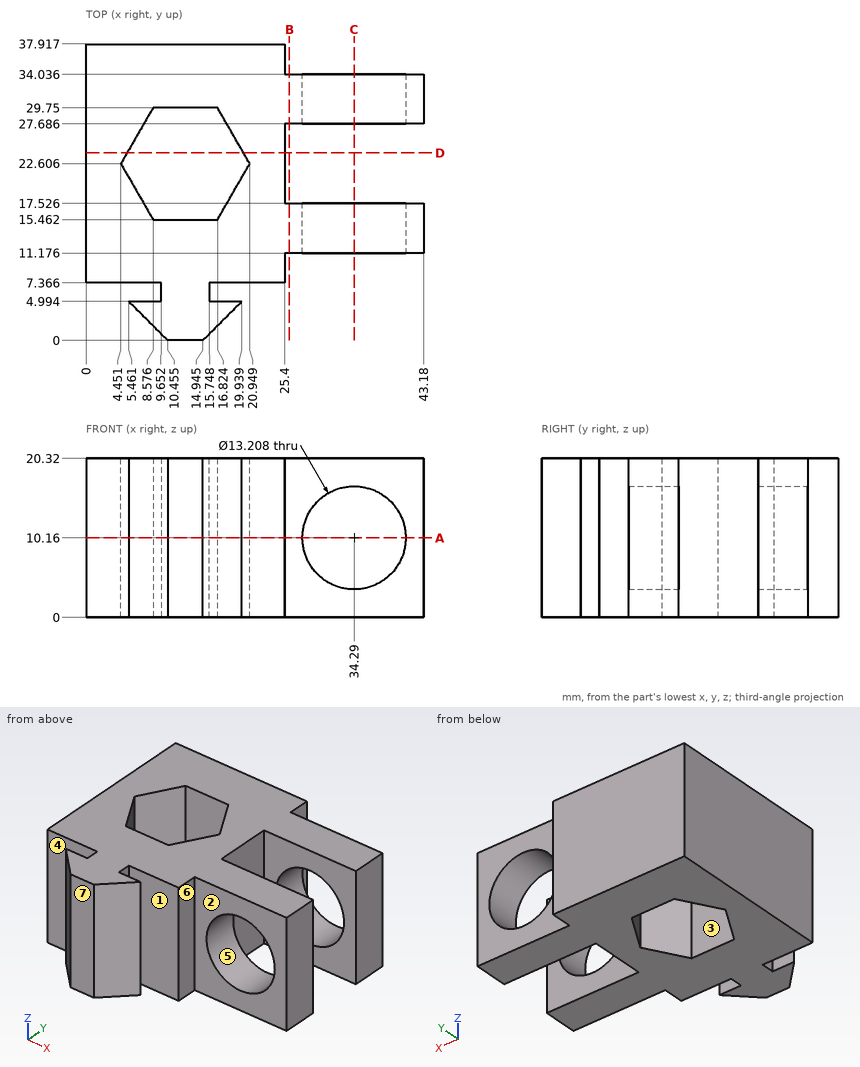
Here's the drawing with two shaded views (mm, measured from the low corner). I have some questions. A direction names the side the tool comes from. Give positions to 0.01 mm unless a question says otherwise; leave off trailing zeros. Order: outer loops, then holes, each group sorted by start corner. A loop starts at its lowest first (then second) coordinate and runs counter-clockwise, first axis right, second up. Notation, with made-up numbers: M -19.5,37 L 33.5,37 A21 ccw 33.5,44 Z; hole C 15.25,11.25 d5. An arc over 180 degrees is marked long. Answer as a JSON object with one key per item and string values. Group by question number.
1) Suppose I cut it at B-B, the plane x = 26. Write out the boundary of the cut face in (y, z).
2) Suppose I cut it at C-C, the plane x = 34.29. Write out the boundary of the cut face in (y, z).
3) We'd pull the mould along X, two halves only. Please class the marked faces 5, 6 and 7: pulls with the +X half, pulls with the -X half, needs draft (parallel to the pull), parting line crosses it, or undercut.
4) Suppose I cut it at D-D, the plane y = 24. Write out the boundary of the cut face in (x, z), plus the area to 3 significant figures.
5) I'm going to push flat-ended pins straight in: pin 1 Ø4 at (y, z) = (8.5, 9.5) entering from +X; pin 2 Ø10 at (x, z) = (33.5, 16) entering from -Y; pin 3 Ø10 at (y, z) = (22.5, 17) entering from -X; pin 4 Ø1.9 at (y, z) = (6, 7.5) entering from -X. Where does each tip first touch, or does it pass through?
6) Please list where these lines run through material, in increasing order: L1, parallel to Z at x = 34.29, y = 31.75; L2, parallel to Y at x = 6, z = 15.5 (1 decimal); L3, parallel to Y at x = 8.5, z = 17 (1 decimal). Write a range as [from, to].
7) On a 3-axis mill with a long thin cutter (end or side, diameter ignored), from which of +Z, -Z, +X, -X, +Y, -Y can I reach the whole of each face in a straight line? I mean the marked faces 1, 2, 3 and 4. Say none if no direction works.
8) Suppose I cut it at A-A, the plane z = 10.16. Count the separate pieces of the cut face and the enclosed holes in it, plus the area to 3 significant figures.
Results found:
{
 "1": {"outline": "M 11.18,0 L 17.53,0 L 17.53,20.32 L 11.18,20.32 Z; M 27.69,0 L 34.04,0 L 34.04,20.32 L 27.69,20.32 Z"},
 "2": {"outline": "M 11.18,0 L 17.53,0 L 17.53,3.56 L 11.18,3.56 Z; M 11.18,16.76 L 17.53,16.76 L 17.53,20.32 L 11.18,20.32 Z; M 27.69,0 L 34.04,0 L 34.04,3.56 L 27.69,3.56 Z; M 27.69,16.76 L 34.04,16.76 L 34.04,20.32 L 27.69,20.32 Z"},
 "3": {"face 5": "undercut", "face 6": "pulls with the +X half", "face 7": "needs draft"},
 "4": {"outline": "M 0,0 L 5.26,0 L 5.26,20.32 L 0,20.32 Z; M 20.14,0 L 25.4,0 L 25.4,20.32 L 20.14,20.32 Z", "area": "214 mm²"},
 "5": {"pin 1": "x = 25.4", "pin 2": "y = 11.18", "pin 3": "x = 0", "pin 4": "x = 9.65"},
 "6": {"L1": "[0, 3.56], [16.76, 20.32]", "L2": "[4.5, 5], [7.4, 19.9], [25.3, 37.9]", "L3": "[2, 5], [7.4, 15.6], [29.6, 37.9]"},
 "7": {"face 1": "+Z, -Z, +X", "face 2": "+Z, -Z, +X, -Y", "face 3": "+Z, -Z", "face 4": "+Z, -Z, -X"},
 "8": {"separate pieces": "3", "enclosed holes": "1", "area": "719 mm²"}
}
